from build123d import *

# Parameters (mm, degrees)
F0_W     = 76.2
F0_H     = 76.2
F1_DEPTH = 2.3622
F2_W     = 25.4
F2_H     = 2.3622
F3_DEPTH = 2.3632
F4_W     = 2.3622
F4_H     = 35.7378
F5_DEPTH = 25.4
F6_W     = 12.7
F6_H     = 2.286
F6_H_2   = 2.3622
F7_DEPTH = 25.4


# Not quite as in the source:
# - a pattern or mirror of a feature is missing from the dataset's text; its kind, count and spacing are read off the source's solid


with BuildPart() as f1:
    # F0 (on Front) → F1 (new body)
    with BuildSketch(Plane.XZ):
        Rectangle(F0_W, F0_H)
    extrude(amount=F1_DEPTH)

    # F2 (on face) → F3 (cut, through all)
    with BuildSketch(Plane.XZ.offset(2.3622)):
        with Locations((-25.4, 36.9189)):
            Rectangle(F2_W, F2_H)
        with Locations((25.4, 36.9189)):
            Rectangle(F2_W, F2_H)
    f3 = extrude(amount=-F3_DEPTH, mode=Mode.SUBTRACT)

    # F3_copies: F3 across plane
    add(f3.mirror(Plane(origin=(0, 0, 0), x_dir=(-1, 0, 0), z_dir=(0, 0, -1))), mode=Mode.SUBTRACT)

    # F4 (on face) → F5 (cut)
    with BuildSketch(Plane.XZ.offset(2.3622)):
        with Locations((-36.9189, 17.8689)):
            Rectangle(F4_W, F4_H)
        with Locations((36.9189, -17.8689)):
            Rectangle(F4_W, F4_H)
    extrude(amount=-F5_DEPTH, mode=Mode.SUBTRACT)

    # F6 (on face) → F7 (cut)
    with BuildSketch(Plane.XZ.offset(2.3622)):
        with Locations((0, 20.2311)):
            Rectangle(F6_W, F6_H)
        with Locations((0, 7.5311)):
            Rectangle(F6_W, F6_H_2)
    extrude(amount=-F7_DEPTH, mode=Mode.SUBTRACT)


solid = f1.part
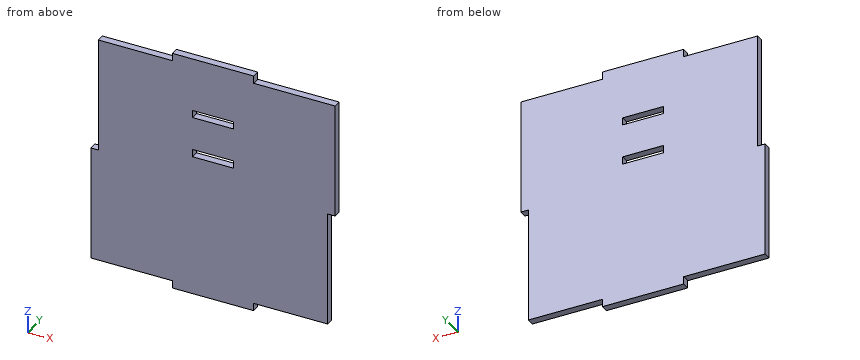
The listing builds one solid part. Answer for the finished solid, in the listing's coordinates (mm). Coordinates: 2 decimals unless noted, no trailing zeros. Write each loop counter-clockwise with the first axis right and the second up, starting at its lowest first coordinate (ties: lowest second). Pieces come first, ordered by that corner, then holes. Notation, with made-up numbers: M -35.75,79 L -9.75,79 A31 cw -9.75,114 Z; hole C 44.5,68 d7. An arc over 180 degrees is marked long. Write each question's results on one line, items separated by ' | '.
Item 1: The part is cut by section D-D on z = -22. Determine the outline of the cut face in (x, y), and give its area (3 significant figures).
Answer below:
outline: M -38.1,-2.36 L 35.74,-2.36 L 35.74,0 L -38.1,0 Z | area: 174 mm2
Item 2: Consider probe 1 along Z at (x, y) = (5, -0.8); probe 2 along X at (y, z) = (-2.1, -3.5); probe 3 along Z at (x, y) = (-31, -0.15). Determine where each line is inside the solid, lowest interval first. Write a range as [from, to].
Answer below:
probe 1: [-38.1, 6.35], [8.71, 19.09], [21.37, 38.1] | probe 2: [-38.1, 35.74] | probe 3: [-35.74, 35.74]
Item 3: The part is cut by section A-A on y = -1.4. Determine the outline of the cut face in (x, z).
Answer below:
outline: M -38.1,-35.74 L -12.7,-35.74 L -12.7,-38.1 L 12.7,-38.1 L 12.7,-35.74 L 35.74,-35.74 L 35.74,0 L 38.1,0 L 38.1,35.74 L 12.7,35.74 L 12.7,38.1 L -12.7,38.1 L -12.7,35.74 L -35.74,35.74 L -35.74,0 L -38.1,0 Z; hole M -6.35,6.35 L 6.35,6.35 L 6.35,8.71 L -6.35,8.71 Z; hole M -6.35,19.09 L 6.35,19.09 L 6.35,21.37 L -6.35,21.37 Z
Item 4: The part is cut by section B-B on x = -4.5. Determine the outline of the cut face in (y, z).
Answer below:
outline: M -2.36,-38.1 L 0,-38.1 L 0,6.35 L -2.36,6.35 Z; M -2.36,8.71 L 0,8.71 L 0,19.09 L -2.36,19.09 Z; M -2.36,21.37 L 0,21.37 L 0,38.1 L -2.36,38.1 Z
Item 5: The part is cut by section C-C on x = -14.5. Determine the outline of the cut face in (y, z), and give its area (3 significant figures).
Answer below:
outline: M -2.36,-35.74 L 0,-35.74 L 0,35.74 L -2.36,35.74 Z | area: 169 mm2
Item 6: Given P1, Ø1.1, axis at y = -1.5, z = 20, coming from the -X side; P2, Ø0.7, axis at y = -1.5, z = -22, coming from the +X side; P3, Ø1.2, axis at x = -37.5, y = -1.5, coming from the +Z side, each flat-ended and moving along its own axis, determine where each tip first touches the part or whether it passes through.
Answer below:
P1: x = -35.74 | P2: x = 35.74 | P3: z = 0
